```python
from build123d import *

# Parameters (mm, degrees)
SKETCH1_R          = 10
EXTRUDE1_DEPTH     = 2.4
SKETCH2_R          = 8.8
EXTRUDE2_DEPTH     = 3.2
FILLET1_R          = 0.8
FILLET2_R          = 0.15
FILLET3_R          = 0.45
SKETCH3_R          = 9.2
SKETCH3_R_2        = 8.8
CUT_EXTRUDE2_DEPTH = 0.2
CUT_EXTRUDE2_TAPER = 20


with BuildPart() as part:
    # Sketch1 → Extrude1 (new body)
    with BuildSketch(Plane(origin=(0, 0, 0), x_dir=(1, 0, 0), z_dir=(0, 1, 0))):
        Circle(SKETCH1_R)
    extrude(amount=EXTRUDE1_DEPTH)

    # Sketch2 → Extrude2 (add)
    with BuildSketch(Plane(origin=(0, 0, 0), x_dir=(1, 0, 0), z_dir=(0, 1, 0))):
        Circle(SKETCH2_R)
    extrude(amount=EXTRUDE2_DEPTH)

    # Fillet1
    fillet1_edges = [part.edges().sort_by_distance(p)[0] for p in [
        (-10, 2.4, 0),
    ]]
    fillet(fillet1_edges, radius=FILLET1_R)

    # Fillet2
    fillet2_edges = [part.edges().sort_by_distance(p)[0] for p in [
        (-10, 0, 0),
    ]]
    fillet(fillet2_edges, radius=FILLET2_R)

    # Fillet3
    fillet3_edges = [part.edges().sort_by_distance(p)[0] for p in [
        (-8.8, 3.2, 0),
    ]]
    fillet(fillet3_edges, radius=FILLET3_R)

    # Sketch3 → Cut-Extrude2 (cut)
    with BuildSketch(Plane(origin=(0, 2.4, 0), x_dir=(-1, 0, 0), z_dir=(0, 1, 0))):
        Circle(SKETCH3_R)
        Circle(SKETCH3_R_2, mode=Mode.SUBTRACT)
    extrude(amount=-CUT_EXTRUDE2_DEPTH, taper=CUT_EXTRUDE2_TAPER, mode=Mode.SUBTRACT)


solid = part.part
```
For this review, take the finished solid that the model builds, in its own axes (mm). A direction names the side the tool comes from. Coordinates: 2 decimals unless noted, no trailing zeros. Loops run counter-clockwise (first coordinate to the right, second up) from the corner with the lowest first, then second, coordinate; pieces in that order, holes last.
1. Add section A-A, the plane x = 0. Give the boundary of the cut face in (y, z), then the cut area to 3 significant figures.
2. Add section B-B, the plane y = 0.65. Give the boundary of the cut face in (x, z), then the cut area to 3 significant figures.
3. For line 1 (X direction, y = 0.2, z = 5.5); line 2 (Z direction, x = 1.75, y = 1.05); line 3 (Y direction, x = 1, z = 8.5), list the stretches that pass through material, from the lowest coordinate up.
4. For faces 1 (the cylindrical face through (8.394, 2.573, -2.643)), 2 (the flat face through (0, 3.2, 0)), list the 3-axis set-ups (+Z, -Z, +X, -X, +Y, -Y) from which the entire face can be reached by the end or side of a thin tool; tool diameter is ignored.
5. Insertion check: P1, Ø1.5, axis at x = 8, y = 1, coming from the +Z side; P2, Ø1, axis at x = 1.5, y = 0.5, coming from the +Z side; P3, Ø1.5, axis at y = 0.5, z = 3, coming from the -X side. Each pin has a flat end and moves straight along its axis. Give the tip position at first contact, or say it passes through.
Result:
1. outline: (0, -9.85) arc R0.15 ccw to (0.15, -10) - (1.6, -10) arc R0.8 ccw to (2.4, -9.2) - (2.2, -9.13) - (2.2, -8.87) - (2.4, -8.8) - (2.75, -8.8) arc R0.45 ccw to (3.2, -8.35) - (3.2, 8.35) arc R0.45 ccw to (2.75, 8.8) - (2.4, 8.8) - (2.2, 8.87) - (2.2, 9.13) - (2.4, 9.2) arc R0.8 ccw to (1.6, 10) - (0.15, 10) arc R0.15 ccw to (0, 9.85) - close
1. area: 61.6 mm2
2. outline: circle Ø20 at (0, 0)
2. area: 314 mm2
3. line 1: x = -8.35 to 8.35
3. line 2: z = -9.85 to 9.85
3. line 3: y = 0 to 3.15
4. face 1: +Y
4. face 2: +Z, -Z, +X, -X, +Y
5. P1: stops at z = 6.89
5. P2: stops at z = 9.95
5. P3: stops at x = -9.74
